from build123d import *

# Parameters (mm, degrees)
BOSS_EXTRUDE2_DEPTH = 5.4
BOSS_EXTRUDE3_DEPTH = 60
SKETCH28_R          = 1.6
CUT_EXTRUDE3_DEPTH  = 8.2
SKETCH29_R          = 1.6
CUT_EXTRUDE4_DEPTH  = 8.2
SKETCH30_R          = 1.6
CUT_EXTRUDE5_DEPTH  = 8.2
SKETCH31_R          = 1.6
CUT_EXTRUDE6_DEPTH  = 8.2
CUT_EXTRUDE7_DEPTH  = 50
SKETCH33_R          = 2.5
BOSS_EXTRUDE4_DEPTH = 15.4


with BuildPart() as part:
    # Sketch1 → Boss-Extrude2 (new body)
    with BuildSketch(Plane(origin=(0, 0, 0), x_dir=(1, 0, 0), z_dir=(0, 1, 0))):
        Polygon((-266.076640718, -7.104357828), (-272.301088237, 3.676701524), (-249.238844193, 43.621679945), (-236.789949155, 43.621679945), (-10.515779175, 43.621679945), (1.933115864, 43.621679945), (24.995359908, 3.676701524), (18.770912388, -7.104357828), (-94.366172601, -203.063537251), (-100.590620121, -213.844596604), (-146.715108209, -213.844596604), (-152.939555728, -203.063537251), align=None)
    extrude(amount=BOSS_EXTRUDE2_DEPTH)

    # Sketch25 → Boss-Extrude3 (add)
    with BuildSketch(Plane.XZ):
        Polygon((-272.301088237, -3.676701524), (-249.238844193, -43.621679945), (1.933115864, -43.621679945), (24.995359908, -3.676701524), (-100.590620121, 213.844596604), (-146.715108209, 213.844596604), align=None)
    extrude(amount=BOSS_EXTRUDE3_DEPTH)

    # Sketch28 → Cut-Extrude3 (cut)
    with BuildSketch(Plane(origin=(-202.633757717, 0, 116.990654565), x_dir=(0.499999999999994, 0, 0.8660254037844421), z_dir=(-0.8660254037844421, 0, 0.499999999999994))):
        with Locations((95.888403978, 2.9)):
            Circle(SKETCH28_R)
        with Locations((102.888403978, 2.9)):
            Circle(SKETCH28_R)
    extrude(amount=-CUT_EXTRUDE3_DEPTH, mode=Mode.SUBTRACT)

    # Sketch29 → Cut-Extrude4 (cut)
    with BuildSketch(Plane(origin=(-202.633757717, 0, 116.990654565), x_dir=(0.499999999999994, 0, 0.8660254037844421), z_dir=(-0.8660254037844421, 0, 0.499999999999994))):
        with Locations((-130.385766002, 2.9)):
            Circle(SKETCH29_R)
        with Locations((-123.385766002, 2.9)):
            Circle(SKETCH29_R)
    extrude(amount=-CUT_EXTRUDE4_DEPTH, mode=Mode.SUBTRACT)

    # Sketch30 → Cut-Extrude5 (cut)
    with BuildSketch(Plane(origin=(0, 0, -43.621679945), x_dir=(-1, 0, 0), z_dir=(0, 0, -1))):
        with Locations((233.289949155, 2.9)):
            Circle(SKETCH30_R)
        with Locations((240.289949155, 2.9)):
            Circle(SKETCH30_R)
        with Locations((7.015779175, 2.9)):
            Circle(SKETCH30_R)
        with Locations((14.015779175, 2.9)):
            Circle(SKETCH30_R)
    extrude(amount=-CUT_EXTRUDE5_DEPTH, mode=Mode.SUBTRACT)

    # Sketch31 → Cut-Extrude6 (cut)
    with BuildSketch(Plane(origin=(17.15446147, 0, 9.904132947), x_dir=(0.49999999999999983, 0, -0.8660254037844387), z_dir=(0.8660254037844387, 0, 0.49999999999999983))):
        with Locations((-0.267098163, 2.9)):
            Circle(SKETCH31_R)
        with Locations((6.732901837, 2.9)):
            Circle(SKETCH31_R)
        with Locations((-226.541268142, 2.9)):
            Circle(SKETCH31_R)
        with Locations((-219.541268142, 2.9)):
            Circle(SKETCH31_R)
    extrude(amount=-CUT_EXTRUDE6_DEPTH, mode=Mode.SUBTRACT)

    # Sketch32 → Cut-Extrude7 (cut)
    with BuildSketch(Plane(origin=(0, 5.4, 0), x_dir=(1, 0, 0), z_dir=(0, 1, 0))):
        Polygon((-252.809368412, -30.08394754), (-222.888866427, -12.809337664), (-210.255404543, 9.072460194), (-210.255404543, 43.621679945), (-37.050323786, 43.621679945), (-37.050323786, 9.072460194), (-24.416861903, -12.809337664), (5.503640083, -30.08394754), (-81.098900296, -180.08394754), (-111.019402281, -162.809337664), (-136.286326048, -162.809337664), (-166.206828034, -180.08394754), align=None)
    extrude(amount=-CUT_EXTRUDE7_DEPTH, mode=Mode.SUBTRACT)

    # Sketch33 → Boss-Extrude4 (add)
    # profile 1 of 6: a face of its own
    with BuildSketch(Plane(origin=(0, -44.6, 0), x_dir=(1, 0, 0), z_dir=(0, 1, 0))):
        with BuildLine():
            Line((-57.550882031, 43.621679945), (-47.550882031, 43.621679945))
            Line((-47.550882031, 43.621679945), (-47.550882031, 48.621679945))
            ThreePointArc((-47.550882031, 48.621679945), (-52.550882031, 53.621679945), (-57.550882031, 48.621679945))
            Line((-57.550882031, 48.621679945), (-57.550882031, 43.621679945))
        make_face()
        with Locations(Location((-52.550882031, 48.621679945, 0), (0, 0, 270))):
            Circle(SKETCH33_R, mode=Mode.SUBTRACT)
    # profile 2 of 6: a face of its own
    with BuildSketch(Plane(origin=(0, -44.6, 0), x_dir=(1, 0, 0), z_dir=(0, 1, 0))):
        with BuildLine():
            Line((-189.754846299, 43.621679945), (-189.754846299, 48.621679945))
            ThreePointArc((-189.754846299, 48.621679945), (-194.754846299, 53.621679945), (-199.754846299, 48.621679945))
            Line((-199.754846299, 48.621679945), (-199.754846299, 43.621679945))
            Line((-199.754846299, 43.621679945), (-189.754846299, 43.621679945))
        make_face()
        with Locations(Location((-194.754846299, 48.621679945, 0), (0, 0, 90))):
            Circle(SKETCH33_R, mode=Mode.SUBTRACT)
    # profile 3 of 6: a face of its own
    with BuildSketch(Plane(origin=(0, -44.6, 0), x_dir=(1, 0, 0), z_dir=(0, 1, 0))):
        with BuildLine():
            Line((-242.55908929, -47.837951771), (-247.55908929, -39.177697733))
            Line((-247.55908929, -39.177697733), (-251.889216309, -41.677697733))
            ThreePointArc((-251.889216309, -41.677697733), (-253.719343328, -48.507824752), (-246.889216309, -50.337951771))
            Line((-246.889216309, -50.337951771), (-242.55908929, -47.837951771))
        make_face()
        with Locations(Location((-249.389216309, -46.007824752, 0), (0, 0, 270))):
            Circle(SKETCH33_R, mode=Mode.SUBTRACT)
    # profile 4 of 6: a face of its own
    with BuildSketch(Plane(origin=(0, -44.6, 0), x_dir=(1, 0, 0), z_dir=(0, 1, 0))):
        with BuildLine():
            Line((-176.457107156, -162.329943308), (-180.787234175, -164.829943308))
            ThreePointArc((-180.787234175, -164.829943308), (-182.617361194, -171.660070327), (-175.787234175, -173.490197346))
            Line((-175.787234175, -173.490197346), (-171.457107156, -170.990197346))
            Line((-171.457107156, -170.990197346), (-176.457107156, -162.329943308))
        make_face()
        with Locations(Location((-178.287234175, -169.160070327, 0), (0, 0, 90))):
            Circle(SKETCH33_R, mode=Mode.SUBTRACT)
    # profile 5 of 6: a face of its own
    with BuildSketch(Plane(origin=(0, -44.6, 0), x_dir=(1, 0, 0), z_dir=(0, 1, 0))):
        with BuildLine():
            Line((-70.848621174, -162.329943308), (-75.848621174, -170.990197346))
            Line((-75.848621174, -170.990197346), (-71.518494155, -173.490197346))
            ThreePointArc((-71.518494155, -173.490197346), (-64.688367136, -171.660070327), (-66.518494155, -164.829943308))
            Line((-66.518494155, -164.829943308), (-70.848621174, -162.329943308))
        make_face()
        with Locations(Location((-69.018494155, -169.160070327, 0), (0, 0, 270))):
            Circle(SKETCH33_R, mode=Mode.SUBTRACT)
    # profile 6 of 6: a face of its own
    with BuildSketch(Plane(origin=(0, -44.6, 0), x_dir=(1, 0, 0), z_dir=(0, 1, 0))):
        with BuildLine():
            Line((-4.74663904, -47.837951771), (-0.416512021, -50.337951771))
            ThreePointArc((-0.416512021, -50.337951771), (6.413614998, -48.507824752), (4.583487979, -41.677697733))
            Line((4.583487979, -41.677697733), (0.25336096, -39.177697733))
            Line((0.25336096, -39.177697733), (-4.74663904, -47.837951771))
        make_face()
        with Locations(Location((2.083487979, -46.007824752, 0), (0, 0, 90))):
            Circle(SKETCH33_R, mode=Mode.SUBTRACT)
    extrude(amount=-BOSS_EXTRUDE4_DEPTH)


solid = part.part
The model under review builds one solid part; all positions refer to its coordinate system, in mm. A direction names the side the tool comes from. Round coordinates to 2 decimals unless told otherwise and drop trailing zeros. Loops run counter-clockwise (first coordinate to the right, second up) from the corner with the lowest first, then second, coordinate; pieces in that order, holes last. Notation, with made-up numbers: (65.5, 46) -> (116.5, 46) arc R13 cw to (116.5, 68) -> close; hole circle Ø10 at (4, 80.25). An arc over 180 degrees is marked (long way). One line per question, with ' | ' between items. Start each with the question number.
Item 1: Add section C-C, the plane z = 146. Write out the cut boundary in (x, y).
Item 2: For pin 1 (2.5 mm diameter, centred on x = -234, y = 2.5, fed in from -Z); pin 2 (3 mm diameter, centred on x = -178.29, z = 169.16, fed in from -Y); pin 3 (6 mm diameter, centred on x = -13, y = -49.5, fed in from +Z); pin 4 (17.5 mm diameter, centred on y = -28.5, z = -33, fed in from -X), all flat-tipped, find the tip position at first contact; note any pin that passes through.
Item 3: Draft analysis for pull direction Y (two halves, no side actions). For faces 1 (the face through (-263.587, 2.287, 3.332)), 2 (the face through (-241, 5.4, -7)), 3 (the face through (12.72, 2.97, 9.5)), 4 (the face through (-230, -27, -43.622)), state which applies: +Y half, -Y half, draft (parallel to the pull), parting line (faces both ways), or undercut.
Item 4: Machinability: for faces 5 (the face through (-37.05, -19, -27)), 6 (the face through (-30.82, -19.25, 1.72)), 7 (the face through (-18, -27, -43.622)), which of the approach directions +Z, -Z, +X, -X, +Y, -Y give a long, thin tool a straight path to every point of the face, cutting with its end or side? Answer none if there is none.
Item 5: Add section B-B, the plane z = 72.5. Write out the cut boundary in (x, y), then the cut area to 3 significant figures.
Item 6: Add section A-A, the plane y = -18. Write out the cut boundary in (x, z), then the cut area to 3 significant figures.
Item 7: Wall thickness on line 1 along X through (y, z) = (2, -40); line 2 along Y through (x, z) = (-126.5, 141); line 3 along X through (y, z) = (2.5, -23.5): over which ranges is each line inside the solid? List them lowest first. Write a range as [from, to].
Return value:
1) outline: (-185.89, -60) -> (-61.42, -60) -> (-61.42, -44.6) -> (-185.89, -44.6) -> close
2) pin 1: stops at z = -43.62 | pin 2: passes through | pin 3: stops at z = 67.33 | pin 4: stops at x = -260.42
3) face 1: undercut | face 2: +Y half | face 3: undercut | face 4: draft
4) face 5: +Z, -Z, +Y | face 6: +Z, +Y | face 7: -Z, +X, +Y, -Y
5) outline: (-228.32, -60) -> (-18.99, -60) -> (-18.99, -44.6) -> (-228.32, -44.6) -> close | area: 3,220 mm2
6) outline: (-272.3, -3.68) -> (-249.24, -43.62) -> (-210.26, -43.62) -> (-210.26, -9.07) -> (-222.89, 12.81) -> (-252.81, 30.08) -> close; (-166.21, 180.08) -> (-136.29, 162.81) -> (-111.02, 162.81) -> (-81.1, 180.08) -> (-100.59, 213.84) -> (-146.72, 213.84) -> close; (-37.05, -43.62) -> (1.93, -43.62) -> (25, -3.68) -> (5.5, 30.08) -> (-24.42, 12.81) -> (-37.05, -9.07) -> close | area: 9,510 mm2
7) line 1: x = [-251.33, -241.61], [-238.97, -234.61], [-231.97, -210.26], [-37.05, -15.34], [-12.69, -8.34], [-5.69, 4.02] | line 2: y = [-60, -44.6] | line 3: x = [-260.86, -210.26], [-37.05, 13.55]
